Verification items for this drawing (mm, ordinates from the low corner). Round coordinates to 2 decimals unless told otherwise and drop trailing zeros. Order: outer loops, then holes, each group sorted by start corner. A loop starts at its lowest first (then second) coordinate and runs counter-clockwise, first axis right, second up. Notation, with made-up numbers: (67.5, -32.75) -> (125.5, -32.75) arc R19 ccw to (125.5, -7.75) -> close; hole circle Ø9 at (-7.5, 50). An arc over 180 degrees is marked (long way). Use a Markdown table: item, result. Add a question column.
Item 1: Gauge pin test, flat end, axial feed: pin 1 Ø4 at (y, z) = (2, 126) entering from -X. Record the tip position at first contact, or that the pin passes through.
Item 2: Sectioned sample at A-A, the plane z = 185. Record the cut outline in (x, y), and give its area (3 significant figures).
Item 3: Sectioned sample at B-B, the plane y = 3.5. Record the cut outline in (x, z).
Item 4: Material ranges on probe 1 along X at (y, z) = (0.5, 180); probe 2 along X at (y, z) = (2.25, 157); probe 3 along Z at (x, y) = (30, 1), recorded low to high. Write a range as [from, to].
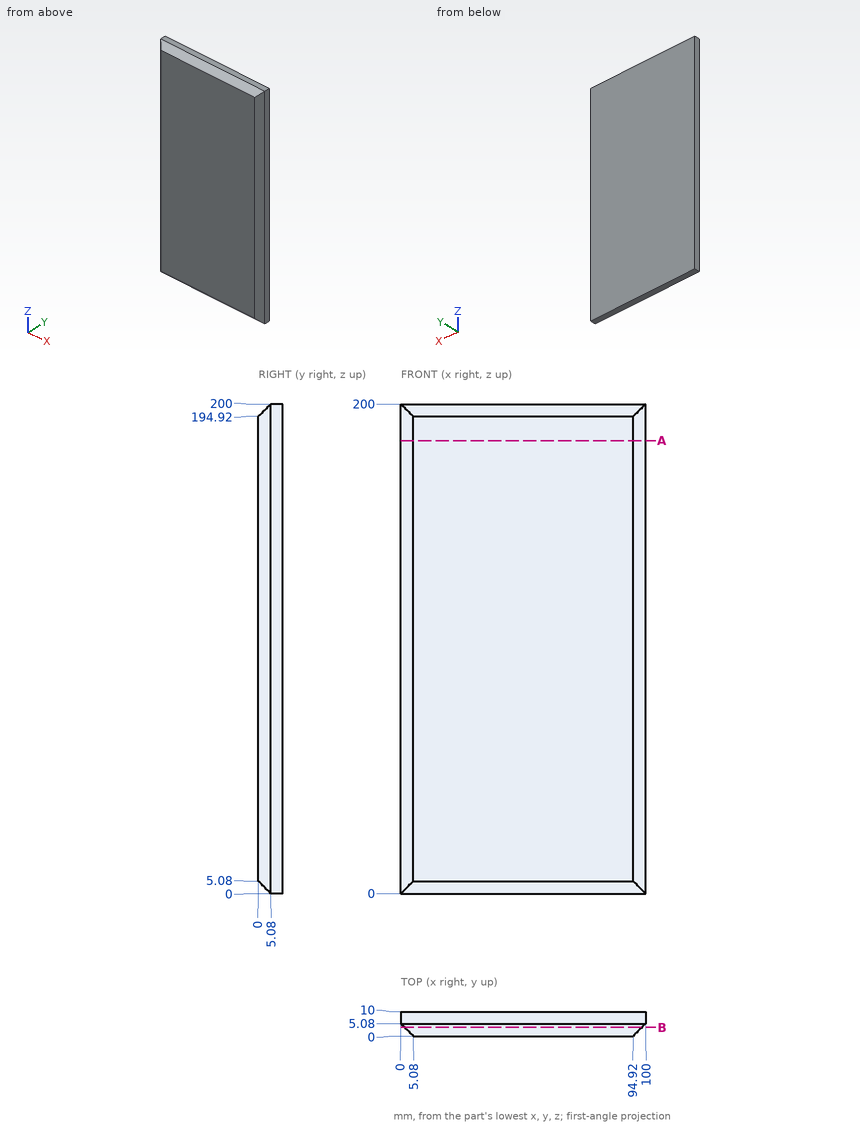
Found:
| question | item | result |
|---|---|---|
| 1 | pin 1 | stops at x = 1.08 |
| 2 | outline | (0, 5.08) -> (5.08, 0) -> (94.92, 0) -> (100, 5.08) -> (100, 10) -> (0, 10) -> close |
| 2 | area | 974 mm2 |
| 3 | outline | (1.58, 1.58) -> (98.42, 1.58) -> (98.42, 198.42) -> (1.58, 198.42) -> close |
| 4 | probe 1 | x = [4.58, 95.42] |
| 4 | probe 2 | x = [2.83, 97.17] |
| 4 | probe 3 | z = [4.08, 195.92] |
